from build123d import *

# Parameters (mm, degrees)
SKETCH_1_W      = 40
SKETCH_1_H      = 40
EXTRUDE_1_DEPTH = 15
SKETCH_2_W      = 25
SKETCH_2_H      = 40
EXTRUDE_2_DEPTH = 15
SKETCH_3_W      = 10
SKETCH_3_H      = 40
EXTRUDE_3_DEPTH = 15


with BuildPart() as part:
    # 草圖1 → 填料-伸長1 (new body)
    with BuildSketch(Plane(origin=(0, 0, 0), x_dir=(1, 0, 0), z_dir=(0, 1, 0))):
        Rectangle(SKETCH_1_W, SKETCH_1_H)
    extrude(amount=EXTRUDE_1_DEPTH)

    # 草圖2 → 填料-伸長2 (add)
    with BuildSketch(Plane(origin=(0, 15, 0), x_dir=(1, 0, 0), z_dir=(0, 1, 0))):
        with Locations((-7.5, 0)):
            Rectangle(SKETCH_2_W, SKETCH_2_H)
    extrude(amount=EXTRUDE_2_DEPTH)

    # 草圖3 → 填料-伸長3 (add)
    with BuildSketch(Plane(origin=(0, 30, 0), x_dir=(1, 0, 0), z_dir=(0, 1, 0))):
        with Locations((-15, 0)):
            Rectangle(SKETCH_3_W, SKETCH_3_H)
    extrude(amount=EXTRUDE_3_DEPTH)


solid = part.part
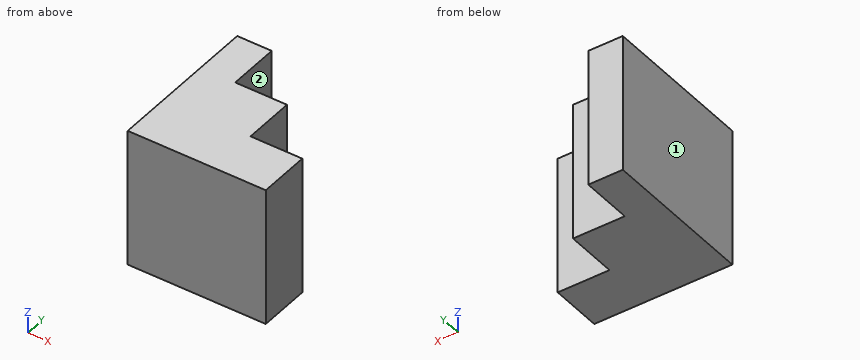
Can you work these out from the model? Positions are in its coordinate system, mm. Face numbers are marked on the shaded views. A direction names the side the tool comes from. Give positions to 0.01 mm unless a question says otherwise; leave off trailing zeros. Order: outer loops, then holes, each group sorted by start corner. A loop starts at its lowest first (then second) coordinate and runs counter-clockwise, first axis right, second up. Notation, with made-up numbers: M 61.5,34 L 71.5,34 A24 ccw 71.5,70 Z; hole C -10.75,2.25 d6. An arc over 180 degrees is marked long. One line per question, with ' | ' between items.
Item 1: Please list where these lines run through material, in increasing order: L1, parallel to X at y = 27, z = -3; L2, parallel to Y at x = 15.5, z = 18; L3, parallel to Y at x = -9, z = 7.
Answer block:
L1: x = -20 to 5 | L2: y = 0 to 15 | L3: y = 0 to 30
Item 2: Suppose I cut it at A-A, the plane z = 12.5. Write out the boundary of the cut face in (x, y), then the cut area to 4 significant figures.
Answer block:
outline: M -20,0 L 20,0 L 20,15 L 5,15 L 5,30 L -10,30 L -10,45 L -20,45 Z | area: 1,125 mm2
Item 3: I'm going to push flat-ended pins straight in: pin 1 Ø4.5 at (x, z) = (0.5, 6) entering from +Y; pin 2 Ø16.5 at (x, z) = (14.5, 8.5) entering from +Y; pin 3 Ø4.5 at (y, z) = (35.5, -3.5) entering from +X. Where does each tip first touch, or does it pass through?
Answer block:
pin 1: stops at y = 30 | pin 2: stops at y = 15 | pin 3: stops at x = -10
Item 4: Suppose I cut it at B-B, the plane x = 7.5. Write out the boundary of the cut face in (y, z), then the cut area to 3 significant figures.
Answer block:
outline: M 0,-20 L 15,-20 L 15,20 L 0,20 Z | area: 600 mm2
Item 5: For the marked faces 1 and 2, which set-ups out of +Z, -Z, +X, -X, +Y, -Y let a thin tool reach every point of the face, with its end or its side?
Answer block:
face 1: +Z, -Z, -X, +Y, -Y | face 2: +Z, -Z, +X, +Y
Item 6: Suppose I cut it at C-C, the plane y = 39. Write out the boundary of the cut face in (x, z), then the cut area to 3 significant figures.
Answer block:
outline: M -20,-20 L -10,-20 L -10,20 L -20,20 Z | area: 400 mm2
